Work out the finished part from the listing and answer in its coordinate system (mm). Round coordinates to 2 decimals unless told otherwise and drop trailing zeros. Loops run counter-clockwise (first coordinate to the right, second up) from the corner with the lowest first, then second, coordinate; pieces in that order, holes last.
Autodesk Inventor part; units mm, degrees
ref_plane "YZ Plane" through (0, 0, 0) normal (1, 0, 0) x (0, 1, 0)
ref_plane "XZ Plane" through (0, 0, 0) normal (0, 1, 0) x (-1, 0, 0)
ref_plane "XY Plane" through (0, 0, 0) normal (0, 0, 1) x (1, 0, 0)
sketch "Sketch1" plane through (0, 0, 0) normal (0, 0, 1) x (1, 0, 0)
  circle A0 centre (0, 0) radius 120
  line L0 (100, 15) -> (220, 15)
  line L1 (220, 15) -> (220, -15)
  line L2 (220, -15) -> (100, -15)
  line L3 (100, -15) -> (100, 15)
  dimension "d0" = 240
  dimension "d1" = 30
  dimension "d2" = 15
  dimension "d3" = 100
  dimension "d4" = 220
extrude "Extrusion1" add sketch "Sketch1" along normal blind 5
fillet "Fillet1" radius 10 4 edges at (119.0588, -15, 2.5) (119.0588, 15, 2.5) (220, -15, 2.5) (220, 15, 2.5)
sketch "Sketch2" plane through (0, 0, 5) normal (0, 0, 1) x (1, 0, 0)
  line L0 (220, -5) -> (220, 5)
  point P0 (0, 0)
  point P1 (135, 0)
  point P2 (205, 0)
  point P3 (220, 0)
  dimension "d8" = 15
  dimension "d9" = 70
hole "Hole1" at (135, 0, 5) at (205, 0, 5) direction (0, 0, -1) diameter 4.496 end through all countersink diameter 8.433 countersink angle 82
sketch "Sketch3" plane through (0, 0, 5) normal (0, 0, 1) x (1, 0, 0)
  point P0 (0, 0)
  point P1 (0, 80)
  dimension "d17" = 80
hole "Hole2" at (0, 80, 5) direction (0, 0, -1) diameter 4.496 end through all countersink diameter 8.433 countersink angle 82
pattern_circular "Circular Pattern1" count 4 over 360 about axis through (0, 0, -10) along (0, 0, 1) of "Hole2"
sketch "Sketch4" plane through (0, 0, 5) normal (0, 0, 1) x (1, 0, 0)
  point P0 (0, 0)
  point P1 (0, 0)
hole "Hole3" at (0, 0, 5) direction (0, 0, -1) diameter 15 end through all
properties part number "Top_Lever Side" material "Wood (Oak)"
1. Determine the mould class of faces 1 (the face through (10, 2, 5)), 2 (the face through (81.75, -1.6, 2.88)), 3 (the face through (207.351, 0.309, 2.877)), 4 (the face through (121.29, -17.22, 2.54)) for opening direction X: +X half, -X half, draft (parallel to the pull), parting line (faces both ways), or undercut.
Answer key:
face 1: draft
face 2: undercut
face 3: undercut
face 4: +X half
2. Find section A-A (x = 170). Write down the section's boundary in (y, z).
Answer key:
outline: (-15, 0) - (15, 0) - (15, 5) - (-15, 5) - close
3. Find section B-B (y = 88.5). Write down the section's boundary in (x, z), then the cut area to 3 significant figures.
Answer key:
outline: (-81.04, 0) - (81.04, 0) - (81.04, 5) - (-81.04, 5) - close
area: 810 mm2
4. Given pin 1 (7 mm diameter, centred on x = 80, y = 0, fed in from -Z); pin 2 (3 mm diameter, centred on x = 28, z = 3.5, fed in from +Y); pin 3 (1 mm diameter, centred on y = 93, z = 1.5, fed in from +X); pin 4 (1 mm diameter, centred on y = -71, z = 3, fed in from +X), each flat-ended and moving along its own axis, determine where each tip first touches the part or whether it passes through.
Answer key:
pin 1: stops at z = 0
pin 2: stops at y = 117.04
pin 3: stops at x = 76.44
pin 4: stops at x = 97.11
5. Consider probe 1 along Y at (x, z) = (205, 1.9); probe 2 along Y at (x, z) = (3, 4.6); probe 3 along Y at (x, z) = (187, 0.3). Determine where each line is inside the solid, lowest interval first.
Answer key:
probe 1: y = -15 to -2.25, 2.25 to 15
probe 2: y = -119.96 to -82.44, -77.56 to -6.87, 6.87 to 77.56, 82.44 to 119.96
probe 3: y = -15 to 15
